Build history of the part. All positions in model axes, mm. A direction names the side the tool comes from. Coordinates: 2 decimals unless noted, no trailing zeros. Write each loop counter-clockwise with the first axis right and the second up, starting at its lowest first coordinate (ties: lowest second). Pieces come first, ordered by that corner, then holes.
```python
from build123d import *

# Parameters (mm, degrees)
SKETCH002_W   = 50
SKETCH002_H   = 50
SKETCH002_W_2 = 10
SKETCH002_H_2 = 10
PAD_DEPTH     = 50


with BuildPart() as part:
    # Sketch002 → Pad (new body, symmetric)
    with BuildSketch(Plane.XZ):
        Rectangle(SKETCH002_W, SKETCH002_H)
        with Locations((-13, 13)):
            Rectangle(SKETCH002_W_2, SKETCH002_H_2, mode=Mode.SUBTRACT)
        with Locations((13, 13)):
            Rectangle(SKETCH002_W_2, SKETCH002_H_2, mode=Mode.SUBTRACT)
        with Locations((13, -13)):
            Rectangle(SKETCH002_W_2, SKETCH002_H_2, mode=Mode.SUBTRACT)
        with Locations((-13, -13)):
            Rectangle(SKETCH002_W_2, SKETCH002_H_2, mode=Mode.SUBTRACT)
    extrude(amount=PAD_DEPTH, both=True)


solid = part.part
```
1. Saw through at A-A on x = 14.5. List the corners of the cut face in (y, z).
Computed values:
outline: (-50, -25) - (50, -25) - (50, -18) - (-50, -18) - close; (-50, -8) - (50, -8) - (50, 8) - (-50, 8) - close; (-50, 18) - (50, 18) - (50, 25) - (-50, 25) - close
2. Mould opens along X. For faces 1 (the face through (-13, -1, -8)), 2 (the face through (0, -1, -25)), 3 (the face through (25, -1, 0)), 4 (the face through (-25, -1, 0)) say: +X half, -X half, draft (parallel to the pull), parting line (faces both ways), or undercut.
Computed values:
face 1: undercut
face 2: draft
face 3: +X half
face 4: -X half
3. Saw through at C-C on y = 0. List the corners of the cut face in (x, z).
Computed values:
outline: (-25, -25) - (25, -25) - (25, 25) - (-25, 25) - close; hole (-18, -18) - (-8, -18) - (-8, -8) - (-18, -8) - close; hole (-18, 8) - (-8, 8) - (-8, 18) - (-18, 18) - close; hole (8, -18) - (18, -18) - (18, -8) - (8, -8) - close; hole (8, 8) - (18, 8) - (18, 18) - (8, 18) - close
4. Saw through at B-B on z = 12. List the corners of the cut face in (x, y), plus the area to 3 significant figures.
Computed values:
outline: (-25, -50) - (-18, -50) - (-18, 50) - (-25, 50) - close; (-8, -50) - (8, -50) - (8, 50) - (-8, 50) - close; (18, -50) - (25, -50) - (25, 50) - (18, 50) - close
area: 3,000 mm2
5. Probe line 1 along Z through (x, y) = (-9, -19.5). List the from-to ranges inside material, lowest first.
Computed values:
line 1: z = -25 to -18, -8 to 8, 18 to 25
6. 3-axis set-ups, long thin cutter, end or side, ignore diameter. For faces 5 (the face through (0, -50, 0)), 6 (the face through (-13, -1, 8)): which of +Z, -Z, +X, -X, +Y, -Y reach the whole face in a straight line?
Computed values:
face 5: +Z, -Z, +X, -X, -Y
face 6: +Y, -Y
